Print and shaded views of the part. All mm, measured from the part's lowest x, y and z. Round coordinates to 2 decimals unless told otherwise and drop trailing zeros. Loops run counter-clockwise (first coordinate to the right, second up) from the corner with the lowest first, then second, coordinate; pieces in that order, holes last. Notation, with made-up numbers: (5, -18.5) - (24, -18.5) arc R32 cw to (24, 17.5) - close; hole circle Ø8 at (37, 28). An arc over 180 degrees is marked (long way). Answer as a JSON object with one key per item and string values.
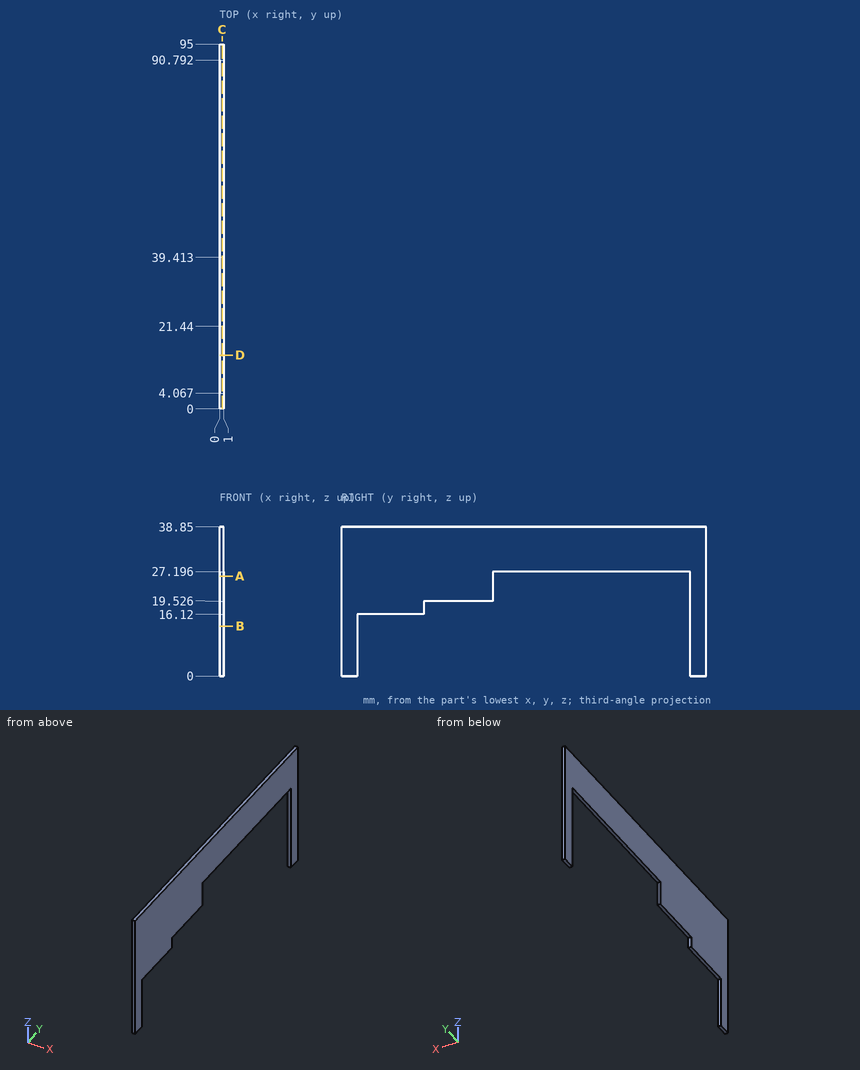
1) Probe probe 1 along Y at (x, z) = (0.5, 17.5); probe 2 along Y at (x, z) = (0.95, 20); probe 3 along Z at (x, y) = (0.85, 8). List the from-to ranges inside material, lowest first.
Values follow:
{"probe 1": "0 to 21.44, 90.79 to 95", "probe 2": "0 to 39.41, 90.79 to 95", "probe 3": "16.12 to 38.85"}
2) Slice it at D-D on y = 14. List the corners of the cut face in (x, z).
Values follow:
{"outline": "(0, 16.12) - (1, 16.12) - (1, 38.85) - (0, 38.85) - close"}
3) Slice it at C-C on x = 0.65. List the corners of the cut face in (y, z).
Values follow:
{"outline": "(0, 0) - (4.07, 0) - (4.07, 16.12) - (21.44, 16.12) - (21.44, 19.53) - (39.41, 19.53) - (39.41, 27.2) - (90.79, 27.2) - (90.79, 0) - (95, 0) - (95, 38.85) - (0, 38.85) - close"}
4) Slice it at B-B on z = 13. List the corners of the cut face in (x, y).
Values follow:
{"outline": "(0, 0) - (1, 0) - (1, 4.07) - (0, 4.07) - close; (0, 90.79) - (1, 90.79) - (1, 95) - (0, 95) - close"}
5) Slice it at A-A on z = 26. List the corners of the cut face in (x, y).
Values follow:
{"outline": "(0, 0) - (1, 0) - (1, 39.41) - (0, 39.41) - close; (0, 90.79) - (1, 90.79) - (1, 95) - (0, 95) - close"}
